Design review of the part built by this model. Coordinates are the model's own, in mm. A direction names the side the tool comes from. Give positions to 0.01 mm unless a question says otherwise; leave off trailing zeros. Loops run counter-clockwise (first coordinate to the right, second up) from the corner with the lowest first, then second, coordinate; pieces in that order, holes last. Notation, with made-up numbers: (62.25, 89.25) -> (91.25, 89.25) arc R18 cw to (91.25, 94.25) -> close; hole circle Ø2 at (46, 41.5). An arc over 180 degrees is marked (long way). Answer as CSV lines item,"result".
from build123d import *

# Parameters (mm, degrees)
SALIENTE_EXTRUIR1_DEPTH = 2.5
CROQUIS3_W              = 38.1
CROQUIS3_H              = 220
SALIENTE_EXTRUIR2_DEPTH = 5
CROQUIS4_W              = 38.1
CROQUIS4_H              = 75
SALIENTE_EXTRUIR3_DEPTH = 5
CROQUIS5_R              = 3
CORTAR_EXTRUIR1_DEPTH   = 5


with BuildPart() as part:
    # Croquis1 → Saliente-Extruir1 (new, symmetric)
    with BuildSketch(Plane(origin=(0, 0, 0), x_dir=(0, 0, -1), z_dir=(1, 0, 0))):
        with BuildLine():
            Line((0, 0), (220, 0))
            Line((220, 0), (220, -16))
            add(Edge.make_bspline(
                [(30, -70), (116.610221718, -10.835054956), (220, -16)],
                knots=[0, 0, 0, 1, 1, 1], degree=2))
            Line((30, -70), (0, -70))
            Line((0, -70), (0, 0))
        make_face()
    extrude(amount=SALIENTE_EXTRUIR1_DEPTH, both=True)

    # Croquis3 → Saliente-Extruir2 (add)
    with BuildSketch(Plane(origin=(0, 0, 0), x_dir=(1, 0, 0), z_dir=(0, 1, 0))):
        with Locations((0, 110)):
            Rectangle(CROQUIS3_W, CROQUIS3_H)
    extrude(amount=SALIENTE_EXTRUIR2_DEPTH)

    # Croquis4 → Saliente-Extruir3 (add)
    with BuildSketch(Plane.XY):
        with Locations((0, -32.5)):
            Rectangle(CROQUIS4_W, CROQUIS4_H)
    extrude(amount=SALIENTE_EXTRUIR3_DEPTH)

    # Croquis5 → Cortar-Extruir1 (cut)
    with BuildSketch(Plane.XY.offset(5)):
        with Locations((-12.645725933, -15.036309881)):
            Circle(CROQUIS5_R)
        with Locations((12.354274067, -15.036309881)):
            Circle(CROQUIS5_R)
        with Locations((-12.595015566, -55.036277737)):
            Circle(CROQUIS5_R)
        with Locations((12.404984434, -55.036277737)):
            Circle(CROQUIS5_R)
    extrude(amount=-CORTAR_EXTRUIR1_DEPTH, mode=Mode.SUBTRACT)


solid = part.part
Q1. The part is to be moulded in two halves that separate along Y. For faces 4 (the flat face through (0, 5, -109)), 5 (the cylindrical face through (9.357, -14.904, 2.535)), 6 (the flat face through (2.5, -27, -87)), say which applies: pulls with the +Y half, pulls with the -Y half, needs draft (parallel to the pull), parting line crosses it, or undercut.
Filled sheet:
face 4,"pulls with the +Y half"
face 5,"undercut"
face 6,"needs draft"
Q2. To check wall thickness, follow probe 1 along Z at (x, y) = (-8, -24.5); probe 2 along X at (y, z) = (-22.5, -50). State the ranges of each line that lie inside material, in increasing order. Write a range as from..to.
Filled sheet:
probe 1,"z = 0..5"
probe 2,"x = -2.5..2.5"
Q3. We need section B-B, the plane x = -12.5. State the section outline as (y, z) points, and give its area (3 significant figures).
Filled sheet:
outline,"(-70, 0) -> (-58.03, 0) -> (-58.03, 5) -> (-70, 5) -> close; (-52.04, 0) -> (-18.03, 0) -> (-18.03, 5) -> (-52.04, 5) -> close; (-12.04, 0) -> (0, 0) -> (0, -220) -> (5, -220) -> (5, 5) -> (-12.04, 5) -> close"
area,"1,420 mm^2"
Q4. For faces 1 (the flat face through (-11, -35, 0)), 2 (the flat face through (11, -35, 0)), 3 (the flat face through (0, 0, -220)), list the 3-axis set-ups (+Z, -Z, +X, -X, +Y, -Y) from which the entire face can be reached by the end or side of a thin tool; tool diameter is ignored.
Filled sheet:
face 1,"-Z, -X, -Y"
face 2,"-Z, +X, -Y"
face 3,"-Z, +X, -X, +Y, -Y"
Q5. Clearance check with flat-ended pins moving along their axes: pin 1 Ø12 at (y, z) = (-14, -93.5) entering from +X; pin 2 Ø13 at (x, z) = (-10.5, -97) entering from -Y; pin 3 Ø9.5 at (x, y) = (12.4, -55.04) entering from -Z. State where each tip first meets the part, or that it passes through.
Filled sheet:
pin 1,"stops at x = 2.5"
pin 2,"stops at y = 0"
pin 3,"stops at z = 0"
Q6. We need section A-A, the plane x = 5.5. State the section outline as (y, z) points.
Filled sheet:
outline,"(-70, 0) -> (0, 0) -> (0, -220) -> (5, -220) -> (5, 5) -> (-70, 5) -> close"
